Geometry check sheet. Reference: the model listing, model coordinates, mm. Face numbers are marked on the shaded views. A direction names the side the tool comes from. Round coordinates to 2 decimals unless told otherwise and drop trailing zeros. Write each loop counter-clockwise with the first axis right and the second up, starting at its lowest first coordinate (ties: lowest second). Pieces come first, ordered by that corner, then holes. Notation, with made-up numbers: M 53,-30.5 L 63,-30.5 A19 cw 63,3.5 Z; hole C 80.25,4 d2. An arc over 180 degrees is marked long. Answer as CSV lines item,"result". Start each with the question number.
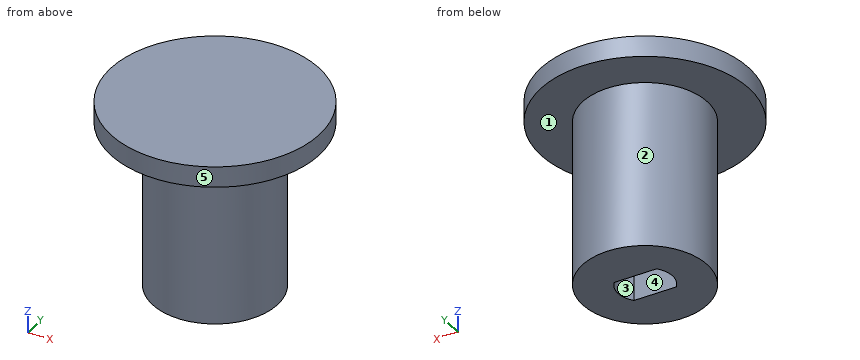
```python
from build123d import *

# Parameters (mm, degrees)
EXTRUDE002_DEPTH  = 7
CYLINDER006_R     = 6
CYLINDER006_DEPTH = 17
CYLINDER_R        = 10
CYLINDER_DEPTH    = 2


with BuildPart() as extrude002:
    # Sketch → Extrude002 (new body)
    with BuildSketch(Plane.XY):
        with BuildLine():
            Line((-2.060088, 8.599999), (2.000001, 8.599999))
            ThreePointArc((2.000001, 5.404159), (2.598634, 7.002079), (2.000001, 8.599999))
            Line((2.000001, 5.404159), (-2.060088, 5.404159))
            ThreePointArc((-2.060088, 8.599999), (-2.651924, 7.002079), (-2.060088, 5.404159))
        make_face()
    extrude(amount=EXTRUDE002_DEPTH)


with BuildPart() as extrude002_1:
    # Extrude002 placement: moved
    add(extrude002.part.moved(Location((-1, 18, 24))))


with BuildPart() as cut015:
    # Cylinder006 → Cylinder006 (new body)
    with BuildSketch(Plane(origin=(-1, 25, 24), x_dir=(1, 0, 0), z_dir=(0, 0, 1))):
        Circle(CYLINDER006_R)
    extrude(amount=CYLINDER006_DEPTH)

    # Cut015: cut Extrude002
    add(extrude002_1.part, mode=Mode.SUBTRACT)


with BuildPart() as obj1:
    # Cylinder → Cylinder (new body)
    with BuildSketch(Plane(origin=(-1, 25, 40), x_dir=(1, 0, 0), z_dir=(0, 0, 1))):
        Circle(CYLINDER_R)
    extrude(amount=CYLINDER_DEPTH)

    # Fusion014: union Cut015
    add(cut015.part)


with BuildPart() as obj1_1:
    # Fusion014 placement: moved
    add(obj1.part.moved(Location((1, -34, 6))))


solid = obj1_1.part
```
1) Section check D-D, the plane y = -13.25. Record the cut outline in (x, z).
2) Scan lines: line 1 (Z direction, x = 4, y = -17.5); line 2 (Y direction, x = -2, z = 31.25); line 3 (Z direction, x = 2.5, y = -9.5). Record each from-to range of solid material in increasing order. Write a range as from..to.
3) Section check A-A, the plane x = 0. Record the cut outline in (y, z).
4) Section check B-B, the plane y = -9. Record the cut outline in (x, z), plus the area to 3 significant figures.
5) Section check C-C, the plane z = 38.5. Record the cut outline in (x, y).
6) Access from +Z, -Z, +X, -X, +Y, -Y to the whole of each face (thin tool, end or side, straight path). Record for the marked faces 4 and 5.
7) Go/stop test with flat-tipped pins: pin 1 (4.5 mm diameter, centred on x = 0, z = 34, fed in from +Y); pin 2 (1.2 mm diameter, centred on x = -0.5, z = 32, fed in from -Y); pin 3 (1.6 mm diameter, centred on x = -0.5, y = -9, fed in from -Z). Record where each tip stops, or that it passes through.
8) Mould release check, pull along X, two halves, no side actions. Record for the marked faces 1, 2 and 3: released by +X, released by -X, zero draft, split by the parting line, or undercut.
Results:
1,outline,"M -9.05,46 L -4.24,46 L -4.24,30 L 4.24,30 L 4.24,46 L 9.05,46 L 9.05,48 L -9.05,48 Z"
2,line 1,"z = 46..48"
2,line 2,"y = -14.66..-10.6, -7.4..-3.34"
2,line 3,"z = 37..48"
3,outline,"M -19,46 L -15,46 L -15,30 L -10.6,30 L -10.6,37 L -7.4,37 L -7.4,30 L -3,30 L -3,46 L 1,46 L 1,48 L -19,48 Z"
4,outline,"M -10,46 L -6,46 L -6,30 L -2.65,30 L -2.65,37 L 2.6,37 L 2.6,30 L 6,30 L 6,46 L 10,46 L 10,48 L -10,48 Z"
4,area,"195 mm^2"
5,outline,"C 0,-9 d12"
6,face 4,"-Z"
6,face 5,"+Z, -Z"
7,pin 1,"stops at y = -3"
7,pin 2,"stops at y = -15"
7,pin 3,"stops at z = 37"
8,face 1,"zero draft"
8,face 2,"split by the parting line"
8,face 3,"undercut"
